Source: CAD feature listing. Evaluate the final solid. Frame: model axes, mm. A direction names the side the tool comes from. Round coordinates to 2 decimals unless told otherwise and drop trailing zeros. Write each loop counter-clockwise with the first axis right and the second up, starting at its lowest first coordinate (ties: lowest second). Pieces come first, ordered by that corner, then holes.
```python
from build123d import *

# Parameters (mm, degrees)
SKETCH1_R           = 10
SKETCH1_R_2         = 2.5
BOSS_EXTRUDE1_DEPTH = 6
SKETCH2_W           = 35
SKETCH2_H           = 6
SKETCH2_W_2         = 6
SKETCH2_H_2         = 35
BOSS_EXTRUDE2_DEPTH = 6
SKETCH3_W           = 20
SKETCH3_H           = 6
SKETCH3_W_2         = 6
SKETCH3_H_2         = 20
BOSS_EXTRUDE3_DEPTH = 7
FILLET1_R           = 10
FILLET2_R           = 3
CHAMFER1_SIZE       = 0.5


with BuildPart() as part:
    # Sketch1 → Boss-Extrude1 (new body)
    # profile 1 of 3: a face of its own
    with BuildSketch(Plane(origin=(0, 0, 0), x_dir=(1, 0, 0), z_dir=(0, 1, 0))):
        with Locations(Location((0, 0, 0), (0, 0, 270))):
            Circle(SKETCH1_R)
        Circle(SKETCH1_R_2, mode=Mode.SUBTRACT)
    # profile 2 of 3: a face of its own
    with BuildSketch(Plane(origin=(0, 0, 0), x_dir=(1, 0, 0), z_dir=(0, 1, 0))):
        with BuildLine():
            ThreePointArc((2.036541185, 1.45), (0, 2.5), (-2.036541185, 1.45))
            Line((-2.036541185, 1.45), (2.036541185, 1.45))
        make_face()
    # profile 3 of 3: a face of its own
    with BuildSketch(Plane(origin=(0, 0, 0), x_dir=(1, 0, 0), z_dir=(0, 1, 0))):
        with BuildLine():
            Line((2.036541185, -1.45), (-2.036541185, -1.45))
            ThreePointArc((-2.036541185, -1.45), (0, -2.5), (2.036541185, -1.45))
        make_face()
    extrude(amount=BOSS_EXTRUDE1_DEPTH)

    # Sketch2 → Boss-Extrude2 (add)
    with BuildSketch(Plane(origin=(0, 6, 0), x_dir=(1, 0, 0), z_dir=(0, 1, 0))):
        with Locations((27.039392014, 0)):
            Rectangle(SKETCH2_W, SKETCH2_H)
        with Locations((0, 27.039392014)):
            Rectangle(SKETCH2_W_2, SKETCH2_H_2)
        with Locations((0, -27.039392014)):
            Rectangle(SKETCH2_W_2, SKETCH2_H_2)
        with Locations((-27.039392014, 0)):
            Rectangle(SKETCH2_W, SKETCH2_H)
    extrude(amount=-BOSS_EXTRUDE2_DEPTH)

    # Sketch3 → Boss-Extrude3 (add)
    with BuildSketch(Plane(origin=(0, 6, 0), x_dir=(1, 0, 0), z_dir=(0, 1, 0))):
        with Locations((-34.539392014, 0)):
            Rectangle(SKETCH3_W, SKETCH3_H)
        with Locations((0, 34.539392014)):
            Rectangle(SKETCH3_W_2, SKETCH3_H_2)
        with Locations((34.539392014, 0)):
            Rectangle(SKETCH3_W, SKETCH3_H)
        with Locations((0, -34.539392014)):
            Rectangle(SKETCH3_W_2, SKETCH3_H_2)
    extrude(amount=BOSS_EXTRUDE3_DEPTH)

    # Fillet1
    fillet1_edges = [part.edges().sort_by_distance(p)[0] for p in [
        (-3, 3, -9.539392014),
        (3, 3, -9.539392014),
        (9.539392014, 3, -3),
        (9.539392014, 3, 3),
        (3, 3, 9.539392014),
        (-3, 3, 9.539392014),
        (-9.539392014, 3, 3),
        (-9.539392014, 3, -3),
    ]]
    fillet(fillet1_edges, radius=FILLET1_R)

    # Fillet2
    fillet2_edges = [part.edges().sort_by_distance(p)[0] for p in [
        (44.539392014, 6.5, -3),
        (44.539392014, 6.5, 3),
        (3, 6.5, 44.539392014),
        (-3, 6.5, 44.539392014),
        (-44.539392014, 6.5, 3),
        (-44.539392014, 6.5, -3),
        (3, 6.5, -44.539392014),
        (-3, 6.5, -44.539392014),
    ]]
    fillet(fillet2_edges, radius=FILLET2_R - 0.0001)  # a hair under: the kernel refuses the full size

    # Chamfer1
    chamfer1_edges = [part.edges().sort_by_distance(p)[0] for p in [
        (19.869038084, 6, -3),
        (24.539392014, 6, 0),
        (24.539392014, 9.5, -3),
        (24.539392014, 9.5, 3),
        (33.039442014, 13, 3),
        (0, 6, 1.45),
        (3, 6, 19.869038084),
        (0, 6, 24.539392014),
        (3, 9.5, 24.539392014),
        (-3, 9.5, 24.539392014),
        (-3, 13, 33.039442014),
        (28.369088084, 0, -3),
        (7.071067812, 6, -7.071067812),
        (7.071067812, 0, -7.071067812),
        (3, 6, -19.869038084),
        (-3, 0, -28.369088084),
        (-7.071067812, 0, -7.071067812),
        (-7.071067812, 6, -7.071067812),
        (-19.869038084, 6, -3),
        (-28.369088084, 0, 3),
        (-7.071067812, 6, 7.071067812),
        (-7.071067812, 0, 7.071067812),
        (-3, 6, 19.869038084),
        (3, 0, 28.369088084),
        (7.071067812, 6, 7.071067812),
        (7.071067812, 0, 7.071067812),
        (19.869038084, 6, 3),
        (11.015384021, 6, -3.917048938),
        (11.015384021, 0, -3.917048938),
        (3.917048938, 6, -11.015384021),
        (3.917048938, 0, -11.015384021),
        (-3.917048938, 6, -11.015384021),
        (-3.917048938, 0, -11.015384021),
        (-2.5, 6, 0),
        (-11.015384021, 6, -3.917048938),
        (-11.015384021, 0, -3.917048938),
        (-11.015384021, 6, 3.917048938),
        (-11.015384021, 0, 3.917048938),
        (-3.917048938, 6, 11.015384021),
        (-3.917048938, 0, 11.015384021),
        (3.917048938, 6, 11.015384021),
        (3.917048938, 0, 11.015384021),
        (11.015384021, 6, 3.917048938),
        (11.015384021, 0, 3.917048938),
        (0, 6, -1.45),
        (33.039442014, 13, -3),
        (43.660741647, 13, 2.121349633),
        (43.660741647, 13, -2.121349633),
        (-28.369088084, 0, -3),
        (3, 0, -28.369088084),
        (28.369088084, 0, 3),
        (-3, 0, 28.369088084),
        (-2.121349633, 0, -43.660741647),
        (2.121349633, 0, -43.660741647),
        (-43.660741647, 0, -2.121349633),
        (-43.660741647, 0, 2.121349633),
        (-2.121349633, 0, 43.660741647),
        (2.121349633, 0, 43.660741647),
        (43.660741647, 0, 2.121349633),
        (43.660741647, 0, -2.121349633),
        (3, 13, 33.039442014),
        (-2.121349633, 13, 43.660741647),
        (2.121349633, 13, 43.660741647),
        (-33.039442014, 13, 3),
        (-43.660741647, 13, -2.121349633),
        (-43.660741647, 13, 2.121349633),
        (-3, 13, -33.039442014),
        (-2.121349633, 13, -43.660741647),
        (2.121349633, 13, -43.660741647),
        (2.5, 6, 0),
        (0, 0, -1.45),
        (-2.5, 0, 0),
        (0, 0, 1.45),
        (-19.869038084, 6, 3),
        (-24.539392014, 6, 0),
        (-24.539392014, 9.5, 3),
        (-24.539392014, 9.5, -3),
        (2.5, 0, 0),
        (-24.539392014, 13, 0),
        (-33.039442014, 13, -3),
        (-3, 6, -19.869038084),
        (0, 6, -24.539392014),
        (-3, 9.5, -24.539392014),
        (3, 9.5, -24.539392014),
        (3, 13, -33.039442014),
    ]]
    chamfer(chamfer1_edges, length=CHAMFER1_SIZE)


solid = part.part
```
Q1. Pin query (flat end, axial travel): P1, Ø3.5, axis at y = 8, z = 34, coming from the -X side; P2, Ø1.5, axis at x = -1, y = 10, coming from the +Z side; P3, Ø6, axis at x = -32, y = 5, coming from the +Z side. Return the tip coordinate at first contact, or that it passes through.
Q2. Section query A-A, the plane y = 7.75. Give the number of separate pieces and of enclosed holes in the cut face, and give its area (3 significant figures).
Q3. Mould query, pull axis Z, two halves, no side actions, for faces 1 (the face through (0, 10, -24.539)), 2 (the face through (2.5, 3, 0)), 3 (the face through (-43.64, 6.58, 2.14)), 4 (the face through (0, 0, 3)). Classes: pulls with the +Z half, pulls with the -Z half, needs draft (parallel to the pull), parting line crosses it, or undercut.
Q4. Section query C-C, the plane z = 33. Output: boundary loops of the cut face in (x, y).
Q5. Line query: line 1 (Z direction, x = -33, y = 11); line 2 (Y direction, x = -4, z = -6). Output: solid intervals per line, ascending.
Q6. Section query B-B, the plane x = -36. Output: boundary loops of the cut face in (y, z).
Q7. Set-up query: faces 5 (the face through (-31, 6, -3)), 6 (the face through (-24.539, 9, 0)), 7 (the face through (-3, 7, 31)), 8 (the face through (0, 3, -1.45)). Return all of +Z, -Z, +X, -X, +Y, -Y with unobstructed straight access to the full face (end or side cutting, diameter ignored); none if empty.
Filled in:
1. P1: stops at x = -3
1. P2: stops at z = 44.53
1. P3: stops at z = 3
2. separate pieces: 4
2. enclosed holes: 0
2. area: 464 mm2
3. face 1: undercut
3. face 2: undercut
3. face 3: pulls with the +Z half
3. face 4: needs draft
4. outline: (-3, 0.5) - (-2.5, 0) - (2.5, 0) - (3, 0.5) - (3, 12.5) - (2.5, 13) - (-2.5, 13) - (-3, 12.5) - close
5. line 1: z = -3 to 3
5. line 2: y = 0 to 6
6. outline: (0, -2.5) - (0.5, -3) - (12.5, -3) - (13, -2.5) - (13, 2.5) - (12.5, 3) - (0.5, 3) - (0, 2.5) - close
7. face 5: -Z, -X, +Y, -Y
7. face 6: +Z, -Z, +Y
7. face 7: +Z, -X, +Y, -Y
7. face 8: +Y, -Y
